Input: dimensioned drawing with shaded views. Units: mm. Origin: part minimum x, y, z. A direction names the side the tool comes from. Give positions to 0.01 mm unless a question says otherwise; leave off trailing zeros. Loops run counter-clockwise (first coordinate to the right, second up) from the corner with the lowest first, then second, coordinate; pieces in that order, holes last.
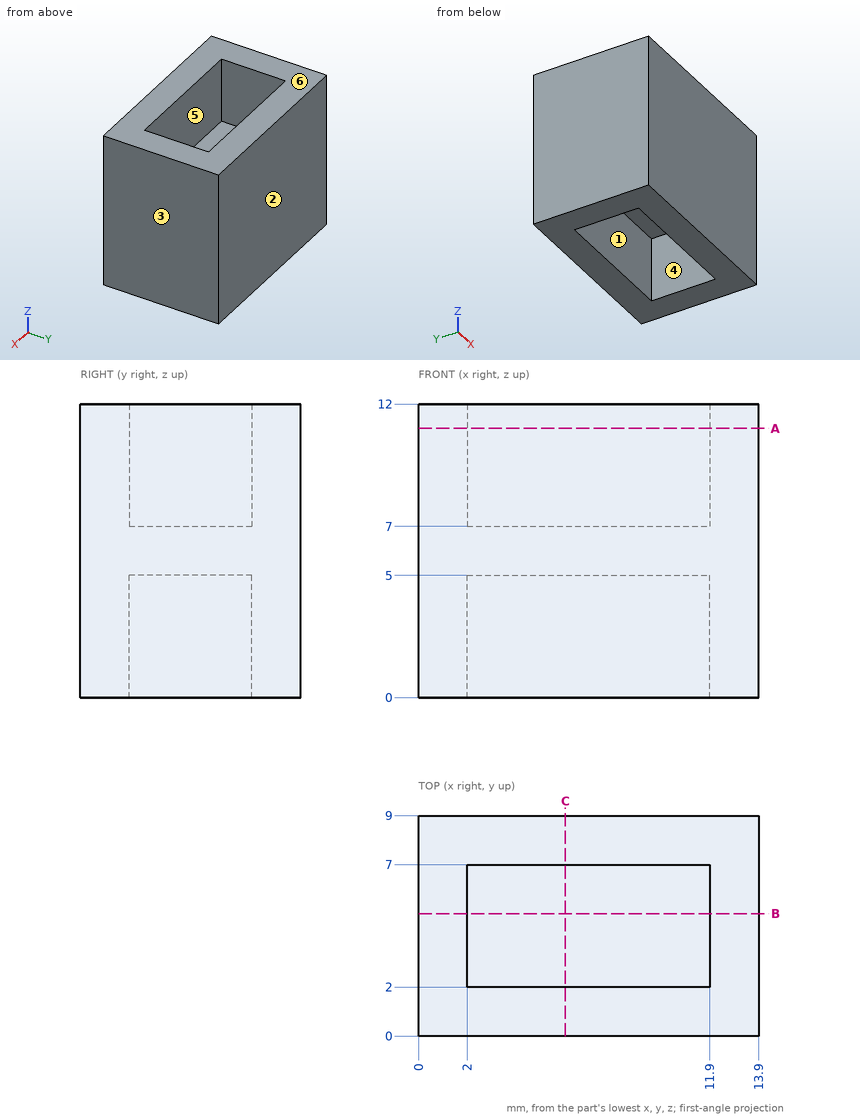
(1) Mould query, pull axis Y, two halves, no side actions, for the marked faces 1, 2 and 3. Classes: pulls with the +Y half, pulls with the -Y half, needs draft (parallel to the pull), parting line crosses it, or undercut.
A:
face 1: undercut
face 2: pulls with the +Y half
face 3: needs draft
(2) Ray query, line 1 along X through (y, z) = (4, 10); line 2 along Y through (x, z) = (9.5, 8.75); line 3 along Z through (x, y) = (3.75, 4). Return the intervals inside material, ascending.
A:
line 1: x = 0 to 2, 11.9 to 13.9
line 2: y = 0 to 2, 7 to 9
line 3: z = 5 to 7
(3) Reachability of the marked faces 4, 5 and 6 from +Z, -Z, +X, -X, +Y, -Y: full face, straight path, thin tool, end or side. Return the list, or none.
A:
face 4: -Z
face 5: +Z
face 6: +Z, +X, -X, +Y, -Y
(4) Section B-B, the plane y = 5. Return the cut outline in (x, z), then the cut area to 3 significant figures.
A:
outline: (0, 0) - (2, 0) - (2, 5) - (11.9, 5) - (11.9, 0) - (13.9, 0) - (13.9, 12) - (11.9, 12) - (11.9, 7) - (2, 7) - (2, 12) - (0, 12) - close
area: 67.8 mm2
(5) First-contact query: pin 1 (3 mm diameter, centred on x = 12, y = 2.5, fed in from -Z); pin 2 (1.5 mm diameter, centred on x = 6.5, y = 3.5, fed in from +Z); pin 3 (4 mm diameter, centred on x = 7.5, y = 4.5, fed in from -Z). Flat tips, straight axial feed; report the tip coordinate or a pass-through.
A:
pin 1: stops at z = 0
pin 2: stops at z = 7
pin 3: stops at z = 5
(6) Section A-A, the plane z = 11. Return the cut outline in (x, y), then the cut area to 3 significant figures.
A:
outline: (0, 0) - (13.9, 0) - (13.9, 9) - (0, 9) - close; hole (2, 2) - (11.9, 2) - (11.9, 7) - (2, 7) - close
area: 75.6 mm2
(7) Section C-C, the plane x = 6. Return the cut outline in (y, z), then the cut area to 3 significant figures.
A:
outline: (0, 0) - (2, 0) - (2, 5) - (7, 5) - (7, 0) - (9, 0) - (9, 12) - (7, 12) - (7, 7) - (2, 7) - (2, 12) - (0, 12) - close
area: 58.0 mm2
